Can you work these out from the drawing? Everything is in mm from the part's minimum corner. A direction names the side the tool comes from. Round coordinates to 2 decimals unless told otherwise and drop trailing zeros. Write each loop counter-clockwise with the first axis right and the second up, starting at its lowest first coordinate (ties: lowest second). Pieces come first, ordered by that corner, then holes.
Q1. For the marked faces 4, 5, 6 and 7, which set-ups out of +Z, -Z, +X, -X, +Y, -Y let a thin tool reach every point of the face, with its end or its side?
Q2. I'm going to push flat-ended pins straight in: pin 1 Ø11 at (y, z) = (44.5, 12) entering from -X; pin 2 Ø16 at (x, z) = (52.5, 9) entering from -Y; pin 3 Ø16 at (x, y) = (39, 13) entering from +Z; pin 4 Ø3 at (x, y) = (21.5, 14.5) entering from +Z. Where does each tip first touch, or does it pass through?
Q3. If we section it at B-B (y = 36): Please give me the cut outline in (x, z).
Q4. If we section it at D-D (y = 19): Please give me the cut outline in (x, z).
Q5. Please list where these lines run through material, in increasing order: line 1 along X through (y, z) = (10.5, 38); line 2 along Z through (x, y) = (31, 8); line 3 along Y through (x, z) = (34.5, 27.5).
Q6. If we section it at C-C (z = 17): Please give me the cut outline in (x, y).
Q7. If we section it at A-A (x = 57): Please give me the cut outline in (y, z).
Q8. We'd pull the mould along X, two halves only. Please class the marked faces 1, 2 and 3: +X half, -X half, draft (parallel to the pull), parting line (faces both ways), or undercut.
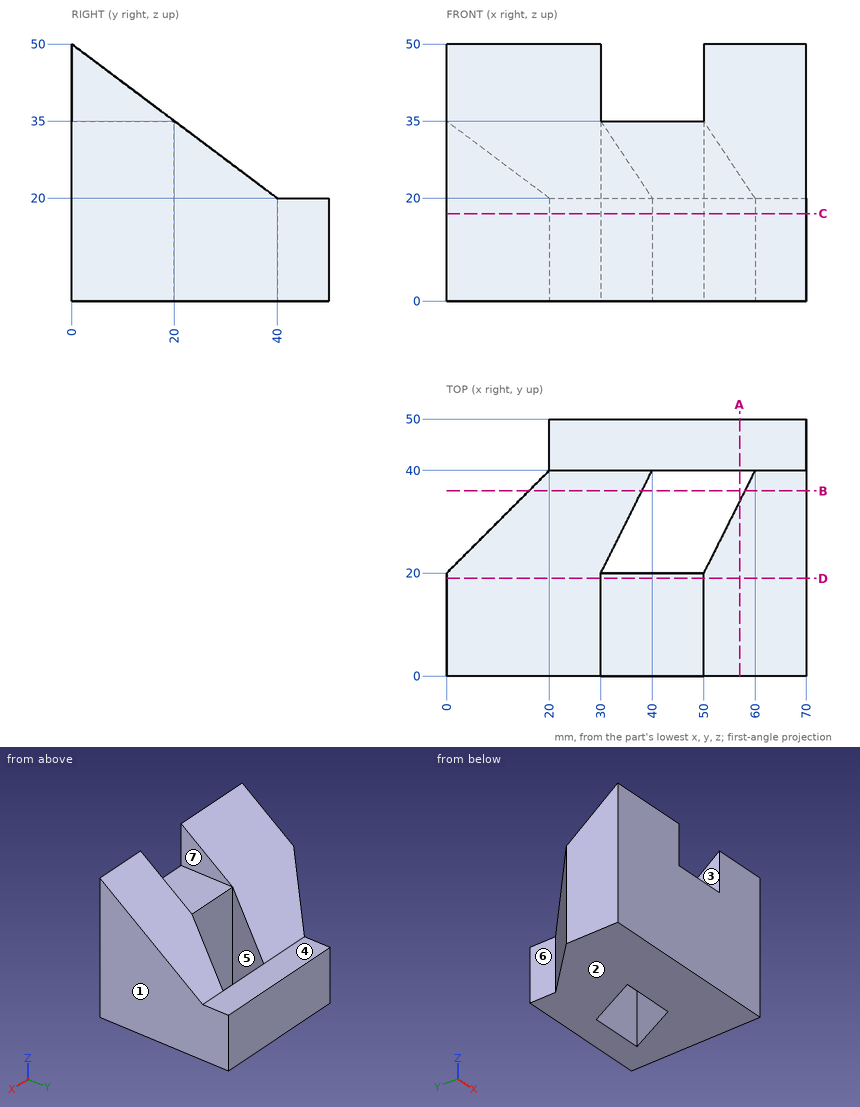
A:
1. face 4: +Z, +X, -X, +Y
1. face 5: +Z, -Z
1. face 6: +Z, -Z, -X, +Y
1. face 7: +Z, +Y, -Y
2. pin 1: stops at x = 19
2. pin 2: stops at y = 0
2. pin 3: stops at z = 35
2. pin 4: stops at z = 40.25
3. outline: (16, 0) - (38, 0) - (38, 23) - (16, 23) - close; (58, 0) - (70, 0) - (70, 23) - (58, 23) - close
4. outline: (0, 0) - (70, 0) - (70, 35.75) - (50, 35.75) - (50, 35) - (30, 35) - (30, 35.75) - (0, 35.75) - close
5. line 1: x = 0 to 30, 50 to 70
5. line 2: z = 0 to 35
5. line 3: y = 0 to 20, 29 to 30
6. outline: (0, 0) - (70, 0) - (70, 50) - (20, 50) - (20, 40) - (0, 20) - close; hole (30, 20) - (50, 20) - (60, 40) - (40, 40) - close
7. outline: (0, 0) - (34, 0) - (34, 24.5) - (0, 50) - close; (40, 0) - (50, 0) - (50, 20) - (40, 20) - close
8. face 1: +X half
8. face 2: draft
8. face 3: undercut
